from build123d import *

# Parameters (mm, degrees)
EXTRUDE_1_DEPTH     = 12
EXTRUDE_2_DEPTH     = 3
CHAMFER_1_SIZE      = 1
SKETCH_3_R          = 2.1
CUT_EXTRUDE_1_DEPTH = 16
CHAMFER_3_SIZE      = 0.5
SKETCH_4_R          = 1.1
CUT_EXTRUDE_2_DEPTH = 44.455844123
SKETCH_5_R          = 1.1
CUT_EXTRUDE_3_DEPTH = 44.455844123
SKETCH_6_R          = 1.1
CUT_EXTRUDE_4_DEPTH = 2.5
CHAMFER_4_SIZE      = 0.5
CHAMFER_5_SIZE      = 0.5
CUT_EXTRUDE_5_DEPTH = 16


with BuildPart() as part:
    # Эскиз1 → Бобышка-Вытянуть1 (new body)
    with BuildSketch(Plane(origin=(0, 0, 0), x_dir=(1, 0, 0), z_dir=(0, 1, 0))):
        Polygon((-7.455844123, 18), (-18, 7.455844123), (-18, -7.455844123), (-7.455844123, -18), (7.455844123, -18), (18, -7.455844123), (18, 7.455844123), (7.455844123, 18), align=None)
        Polygon((-6.420310217, 15.5), (-15.5, 6.420310217), (-15.5, -6.420310217), (-6.420310217, -15.5), (6.420310217, -15.5), (15.5, -6.420310217), (15.5, 6.420310217), (6.420310217, 15.5), align=None, mode=Mode.SUBTRACT)
    extrude(amount=EXTRUDE_1_DEPTH)

    # Эскиз2 → Бобышка-Вытянуть2 (add)
    with BuildSketch(Plane(origin=(0, 12, 0), x_dir=(1, 0, 0), z_dir=(0, 1, 0))):
        Polygon((7.455844123, 18), (-7.455844123, 18), (-18, 7.455844123), (-18, -7.455844123), (-7.455844123, -18), (7.455844123, -18), (18, -7.455844123), (18, 7.455844123), align=None)
    extrude(amount=EXTRUDE_2_DEPTH)

    # Фаска1
    chamfer_1_edges = [part.edges().sort_by_distance(p)[0] for p in [
        (0, 12, -15.5),
        (-10.960155108, 12, -10.960155108),
        (-15.5, 12, 0),
        (-10.960155108, 12, 10.960155108),
        (0, 12, 15.5),
        (10.960155108, 12, 10.960155108),
        (15.5, 12, 0),
        (10.960155108, 12, -10.960155108),
    ]]
    chamfer(chamfer_1_edges, length=CHAMFER_1_SIZE)

    # Эскиз3 → Вырез-Вытянуть1 (cut, through all)
    with BuildSketch(Plane(origin=(0, 15, 0), x_dir=(1, 0, 0), z_dir=(0, 1, 0))):
        Circle(SKETCH_3_R)
        with Locations((-6.363961031, 6.363961031)):
            Circle(SKETCH_3_R)
        with Locations((6.363961031, 6.363961031)):
            Circle(SKETCH_3_R)
        with Locations((6.363961031, -6.363961031)):
            Circle(SKETCH_3_R)
        with Locations((-6.363961031, -6.363961031)):
            Circle(SKETCH_3_R)
    extrude(amount=-CUT_EXTRUDE_1_DEPTH, mode=Mode.SUBTRACT)

    # Фаска3
    chamfer_3_edges = [part.edges().sort_by_distance(p)[0] for p in [
        (-2.1, 12, 0),
        (-8.463961031, 12, -6.363961031),
        (4.263961031, 12, -6.363961031),
        (4.263961031, 12, 6.363961031),
        (-8.463961031, 12, 6.363961031),
    ]]
    chamfer(chamfer_3_edges, length=CHAMFER_3_SIZE)

    # Эскиз4 → Вырез-Вытянуть2 (cut, through all)
    with BuildSketch(Plane(origin=(-12.727922061, 0, 12.727922061), x_dir=(0.707106781, 0, 0.707106781), z_dir=(-0.707106781, 0, 0.707106781))):
        with Locations((0, 6)):
            Circle(SKETCH_4_R)
    extrude(amount=-CUT_EXTRUDE_2_DEPTH, mode=Mode.SUBTRACT)

    # Эскиз5 → Вырез-Вытянуть3 (cut, through all)
    with BuildSketch(Plane(origin=(12.727922061, 0, 12.727922061), x_dir=(0.707106781, 0, -0.707106781), z_dir=(0.707106781, 0, 0.707106781))):
        with Locations((0, 6)):
            Circle(SKETCH_5_R)
    extrude(amount=-CUT_EXTRUDE_3_DEPTH, mode=Mode.SUBTRACT)

    # Эскиз6 → Вырез-Вытянуть4 (cut)
    with BuildSketch(Plane.ZY.offset(18)):
        with Locations((0, 6)):
            Circle(SKETCH_6_R)
    extrude(amount=-CUT_EXTRUDE_4_DEPTH, mode=Mode.SUBTRACT)

    # Фаска4
    chamfer_4_edges = [part.edges().sort_by_distance(p)[0] for p in [
        (11.950104602, 6, -13.505739521),
        (-13.505739521, 6, 11.950104602),
        (-13.505739521, 6, -11.950104602),
        (11.950104602, 6, 13.505739521),
        (-18, 6, -1.1),
    ]]
    chamfer(chamfer_4_edges, length=CHAMFER_4_SIZE)

    # Фаска5
    chamfer_5_edges = [part.edges().sort_by_distance(p)[0] for p in [
        (-2.1, 15, 0),
        (-8.463961031, 15, -6.363961031),
        (4.263961031, 15, -6.363961031),
        (4.263961031, 15, 6.363961031),
        (-8.463961031, 15, 6.363961031),
    ]]
    chamfer(chamfer_5_edges, length=CHAMFER_5_SIZE)

    # Эскиз9 → Вырез-Вытянуть5 (cut, through all)
    with BuildSketch(Plane.XZ):
        Polygon((-8.455844123, 17), (-7.455844123, 18), (7.455844123, 18), (8.455844123, 17), align=None)
    extrude(amount=-CUT_EXTRUDE_5_DEPTH, mode=Mode.SUBTRACT)


solid = part.part
Verification items for the finished model (mm, model axes). A direction names the side the tool comes from. Round coordinates to 2 decimals unless told otherwise and drop trailing zeros. Loops run counter-clockwise (first coordinate to the right, second up) from the corner with the lowest first, then second, coordinate; pieces in that order, holes last. Notation, with made-up numbers: (27.5, 88.5) - (32.5, 88.5) arc R6 ccw to (32.5, 97.5) - close; hole circle Ø1 at (-15, 74). An arc over 180 degrees is marked (long way). Use one line per item in the form item = value.
1. Draft check along X on faces 1 (the flat face through (14.222, 7.395, 11.234)), 2 (the cylindrical face through (-16.51, 6.93, 0.59)), 3 (the flat face through (-0.1, 11.5, 15)). Enter one of: pulls with the +X half, pulls with the -X half, needs draft (parallel to the pull), parting line crosses it, or undercut.
A:
face_1 = pulls with the +X half
face_2 = needs draft
face_3 = undercut
2. Section check C-C on y = 13.75. Record the cut outline in (x, z).
A:
outline = (-18, -7.46) - (-7.46, -18) - (7.46, -18) - (18, -7.46) - (18, 7.46) - (8.46, 17) - (-8.46, 17) - (-18, 7.46) - close; hole circle Ø4.2 at (-6.36, -6.36); hole circle Ø4.2 at (-6.36, 6.36); hole circle Ø4.2 at (0, 0); hole circle Ø4.2 at (6.36, -6.36); hole circle Ø4.2 at (6.36, 6.36)
3. Section check D-D on y = 6. Give the number of separate pieces and of enclosed holes in the cut face, and give its area (3 significant figures).
A:
separate_pieces = 5
enclosed_holes = 0
area = 233 mm²
4. Section check A-A on x = 0. Record the cut outline in (y, z).
A:
outline = (0, -18) - (15, -18) - (15, -2.6) - (14.5, -2.1) - (12.5, -2.1) - (12, -2.6) - (12, -14.5) - (11, -15.5) - (0, -15.5) - close; (0, 15.5) - (11, 15.5) - (12, 14.5) - (12, 2.6) - (12.5, 2.1) - (14.5, 2.1) - (15, 2.6) - (15, 17) - (0, 17) - close
5. Access from +Z, -Z, +X, -X, +Y, -Y to the whole of each face (thin tool, end or side, straight path). Record for faces 4 (the flat face through (0, 7, -18)), 5 (the flat face through (10.9, 4.2, 11.02)).
A:
face_4 = -Z, +X, -X, +Y, -Y
face_5 = -Y
6. Section check B-B on y = 9.75. Record the cut outline in (x, z).
A:
outline = (-18, -7.46) - (-7.46, -18) - (7.46, -18) - (18, -7.46) - (18, 7.46) - (8.46, 17) - (-8.46, 17) - (-18, 7.46) - close; hole (-15.5, -6.42) - (-6.42, -15.5) - (6.42, -15.5) - (15.5, -6.42) - (15.5, 6.42) - (6.42, 15.5) - (-6.42, 15.5) - (-15.5, 6.42) - close
7. Gauge pin test, flat ends, axial feed: pin 1 Ø1 at (x, y) = (12, 11) entering from -Z; pin 2 Ø6.5 at (x, z) = (-6.36, -6.36) entering from -Y; pin 3 Ø1.5 at (x, y) = (-12, 5) entering from +Z; pin 4 Ø10 at (x, z) = (4.5, -8) entering from +Y. Record the tip position at first contact, or that the pin passes through.
A:
pin_1 = -13.96
pin_2 = 12
pin_3 = 14.21
pin_4 = 15
8. Scan lines: probe 1 along Z at (x, y) = (-2, 9.5); probe 2 along X at (y, z) = (8.25, 3.5); probe 3 along X at (y, z) = (13.25, 5.5). Record each from-to range of solid material in increasing order.
A:
probe_1 = -18 to -15.5, 15.5 to 17
probe_2 = -18 to -15.5, 15.5 to 18
probe_3 = -18 to -8.28, -4.45 to 4.45, 8.28 to 18
